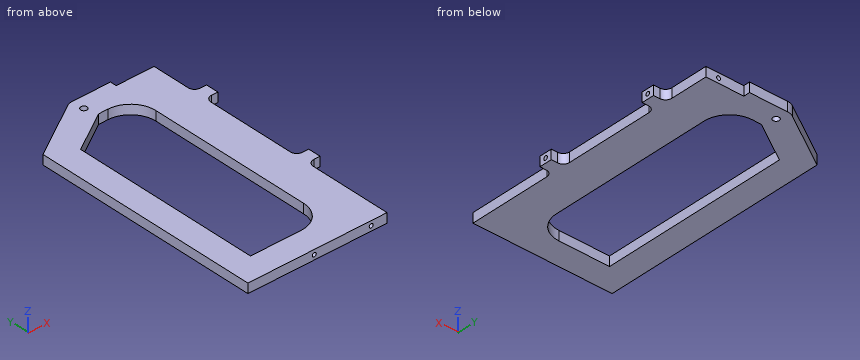
Solid Edge part; units mm, degrees
sketch "Sketch1" plane through (0, 0, 0) normal (0, 0, 1) x (1, 0, 0)
  line L0 (0, 0) -> (0, 266.7)
  line L1 (0, 266.7) -> (88.9, 266.7)
  line L2 (88.9, 266.7) -> (88.9, 0)
  line L3 (88.9, 0) -> (0, 0)
  dimension "D1" = 88.9
extrude "Protrusion1" add sketch "Sketch1" along normal blind 9.525
sketch "Sketch2" plane through (38.1, 127, 9.525) normal (0, 0, 1) x (1, 0, 0)
  line L0 (-38.1, 114.3) -> (-38.1, -101.6)
  line L1 (-38.1, -101.6) -> (12.7, -101.6)
  line L2 (12.7, -101.6) -> (12.7, 114.3)
  line L3 (12.7, 114.3) -> (-38.1, 114.3)
  dimension "D1" = 38.1
  dimension "D2" = 12.7
extrude "Cutout1" cut sketch "Sketch2" against normal through all
hole "Hole_1" at (12.7, 254, 9.525) direction (0, 0, -1) diameter 6.35 end through all
fillet "Round_1" radius 12.7 2 edges at (0, 266.7, 4.7625) (0, 241.3, 4.7625)
fillet "Round_2" radius 25.4 3 edges at (50.8, 241.3, 4.7625) (50.8, 25.4, 4.7625) (0, 25.4, 4.7625)
hole "Hole_9" at (73.025, 0, 4.7625) direction (0, 1, 0) diameter 3.9675 depth 19.05
hole "Hole1" at (15.875, 0, 4.7625) direction (0, 1, 0) diameter 3.9675 depth 19.05
sketch "Sketch3" plane through (44.45, 133.35, 9.525) normal (0, 0, 1) x (1, 0, 0)
  line L0 (44.45, 133.35) -> (44.45, 127)
  line L1 (44.45, 127) -> (6.35, 127)
  line L2 (6.35, 127) -> (6.35, 133.35)
  line L3 (6.35, 133.35) -> (44.45, 133.35)
  dimension "D1" = 6.35
  dimension "D2" = 44.45
extrude "Cutout2" cut sketch "Sketch3" against normal through all
hole "Hole_3" at (76.2, 260.35, 4.7625) direction (0, -1, 0) diameter 3.9675 depth 25.4
sketch "Sketch4" plane through (44.45, 133.35, 9.525) normal (0, 0, 1) x (0, 1, 0)
  line L0 (69.85, -44.45) -> (69.85, -57.15)
  line L1 (69.85, -57.15) -> (82.55, -57.15)
  line L2 (82.55, -57.15) -> (82.55, -44.45)
  line L3 (82.55, -44.45) -> (69.85, -44.45)
  line L4 (-44.45, -44.45) -> (-44.45, -57.15)
  line L5 (-44.45, -57.15) -> (-31.75, -57.15)
  line L6 (-31.75, -57.15) -> (-31.75, -44.45)
  line L7 (-31.75, -44.45) -> (-44.45, -44.45)
  dimension "D1" = 44.45
  dimension "D2" = 44.45
  dimension "D3" = 69.85
  dimension "D4" = 69.85
extrude "ExtrudedProtrusion_2" add sketch "Sketch4" against normal blind 9.525
hole "Hole2" at (101.6, 95.25, 4.7625) direction (-1, 0, 0) diameter 3.9675 depth 25.4
hole "Hole3" at (101.6, 209.55, 4.7625) direction (-1, 0, 0) diameter 3.9675 depth 25.4
fillet "Round_3" radius 6.35 4 edges at (88.9, 88.9, 4.7625) (88.9, 101.6, 4.7625) (88.9, 203.2, 4.7625) (88.9, 215.9, 4.7625)
sketch "Sketch5" plane through (50.8, 133.35, 9.525) normal (0, 0, 1) x (1, 0, 0)
  line L0 (-101.6, 95.6996) -> (-44.8636, 131.3992)
  arc A0 (-38.1, 107.95) -> (-44.8636, 131.3992) centre (-38.1, 120.65) cw
  line L1 (-38.1, 107.95) -> (-34.8078, 107.95)
  line L2 (-76.2, 81.9053) -> (-34.8078, 107.95)
  line L3 (-76.2, -107.95) -> (-76.2, 81.9053)
  line L4 (-25.4, -107.95) -> (-76.2, -107.95)
  line L5 (-25.4, -107.95) -> (-50.8, -133.35)
  line L6 (-50.8, -133.35) -> (-101.6, -133.35)
  line L7 (-101.6, -133.35) -> (-101.6, 95.6996)
extrude "ExtrudedProtrusion_3" add sketch "Sketch5" against normal blind 9.525
properties part number "CHAS-02"
Read the model definition and answer for the solid it produces. Units are mm, in the model's axes. Coordinates: 2 decimals unless noted, no trailing zeros. Write each loop counter-clockwise with the first axis right and the second up, starting at its lowest first coordinate (ties: lowest second). Pieces come first, ordered by that corner, then holes. Notation, with made-up numbers: M -26,7 L 22,7 A25 ccw 22,34 Z; hole C 56.25,10.5 d5. An arc over 180 degrees is marked long. Use a Markdown table: item, result.
Q1. The part is cut by section B-B, the plane y = 254. Write down the section's boundary in (x, z) (1 decimal).
Answer block:
| item | result |
|---|---|
| outline | M -11.1,0 L 9.5,0 L 9.5,9.5 L -11.1,9.5 Z; M 15.9,0 L 88.9,0 L 88.9,9.5 L 15.9,9.5 Z; hole C 76.2,4.8 d4 |
Q2. The part is cut by section C-C, the plane x = 81. Give the number of separate pieces and of enclosed holes in the cut face, then the cut area to 3 significant figures.
Answer block:
| item | result |
|---|---|
| separate pieces | 1 |
| enclosed holes | 2 |
| area | 2,460 mm2 |
Q3. Each of these flat-tipped pins is pushed along its axis until it touches: pin 1 Ø3 at (y, z) = (95.5, 5.5) entering from +X; pin 2 Ø3.5 at (x, z) = (15.88, 4.76) entering from -Y; pin 3 Ø1.9 at (x, z) = (99, 5.5) entering from +Y; pin 4 Ø3 at (y, z) = (95.25, 4.76) entering from +X. Where does it stop, or does it pass through?
Answer block:
| item | result |
|---|---|
| pin 1 | stops at x = 101.6 |
| pin 2 | stops at y = 14.13 |
| pin 3 | stops at y = 215.9 |
| pin 4 | stops at x = 76.2 |
Q4. Straight lines are drawn through the part: L1, parallel to Y at x = 12.7, z = 3 (3 decimals); L2, parallel to X at y = 125, z = 7.5; L3, parallel to Z at x = 76.2, y = 251 (3 decimals). For each, find the intervals that lie inside material, in ascending order. Write a range as [from, to].
Answer block:
| item | result |
|---|---|
| L1 | y = [0, 25.4], [239.228, 250.825], [257.175, 266.7] |
| L2 | x = [-50.8, -25.4], [50.8, 88.9] |
| L3 | z = [0, 2.779], [6.746, 9.525] |
Q5. The part is cut by section A-A, the plane y = 79.5. Write down the section's boundary in (x, z) (3 decimals).
Answer block:
| item | result |
|---|---|
| outline | M -50.8,0 L -25.4,0 L -25.4,9.525 L -50.8,9.525 Z; M 50.8,0 L 88.9,0 L 88.9,9.525 L 50.8,9.525 Z |
